Can you work these out from the model? Positions are in its coordinate system, mm. A direction names the side the tool comes from. Coordinates: 2 decimals unless noted, no trailing zeros. Loops run counter-clockwise (first coordinate to the right, second up) from the corner with the lowest first, then second, coordinate; pieces in that order, holes last. Notation, with made-up numbers: M 55.25,63 L 87.25,63 A21 cw 87.25,96 Z; hole C -12,5.25 d8. An arc over 180 degrees is marked long. Answer as a JSON object with one key per item and string values. Group by question number.
Item 1: Suppose I cut it at C-C (z = -3.5). Write out the boundary of the cut face in (x, y), then the cut area to 3 significant figures.
Item 2: Suppose I cut it at A-A (y = 2.5). Write out the boundary of the cut face in (x, z).
Item 3: Suppose I cut it at B-B (x = 3). Write out the boundary of the cut face in (y, z).
Item 4: We'd pull the mould along Y, two halves only. Please class faces 3 (the flat face through (3, 9, -3)), 4 (the flat face through (6, 5, -3)), 5 (the cylindrical face through (5.49, 2.88, -4.69)): +Y half, -Y half, draft (parallel to the pull), parting line (faces both ways), or undercut.
Item 5: I'm going to push flat-ended pins straight in: pin 1 Ø1.2 at (x, y) = (4, 2) entering from -Z; pin 2 Ø2 at (x, z) = (5.5, -3.5) entering from -Y. Where does each tip first touch, or does it pass through?
Item 6: Which directions (+Z, -Z, +X, -X, +Y, -Y) give clear straight access to the entire face, cutting with the end or side of a thin tool? Please do faces 1 (the flat face through (5, 3, -2)), 2 (the cylindrical face through (1.23, 0.46, -5.02)).
Item 7: Suppose I cut it at D-D (y = 7). Write out the boundary of the cut face in (x, z), then the cut area to 3 significant figures.
Item 8: If I drill on line 1 (X direction, y = 0.75, z = -2.8); line 2 (Y direction, x = 0.5, z = -3.5); line 3 (Z direction, x = 1.2, y = 2.5), over which ranges is the centre line in solid material (lowest first)?
```python
from build123d import *

# Parameters (mm, degrees)
SKETCH1_W           = 5.5
SKETCH1_H           = 9
SKETCH1_R           = 1.25
BOSS_EXTRUDE1_DEPTH = 6
CUT_EXTRUDE3_DEPTH  = 4.5
CUT_EXTRUDE4_REACH  = 14.135
SKETCH5_R           = 1.25
FILLET1_R           = 1.6


with BuildPart() as part:
    # Sketch1 → Boss-Extrude1 (new body)
    with BuildSketch(Plane(origin=(0, 0, 0), x_dir=(0, 0, -1), z_dir=(1, 0, 0))):
        with Locations((2.75, 4.5)):
            Rectangle(SKETCH1_W, SKETCH1_H)
        with Locations((3.5, 2.5)):
            Circle(SKETCH1_R, mode=Mode.SUBTRACT)
    extrude(amount=BOSS_EXTRUDE1_DEPTH)

    # Sketch4 → Cut-Extrude3 (cut)
    with BuildSketch(Plane(origin=(0, 0, -5.5), x_dir=(-1, 0, 0), z_dir=(0, 0, -1))):
        with BuildLine():
            Line((-5, 0), (-5, 4.8))
            ThreePointArc((-5, 4.8), (-3.75, 6.05), (-2.5, 4.8))
            Line((-2.5, 4.8), (-2.5, 0))
            ThreePointArc((-2.5, 0), (-3.75, -1.25), (-5, 0))
        make_face()
    extrude(amount=-CUT_EXTRUDE3_DEPTH, mode=Mode.SUBTRACT)

    # Sketch5 → Cut-Extrude4 (cut, up to next)
    with BuildSketch(Plane.ZY, mode=Mode.PRIVATE) as cut_extrude4_sk1:
        with Locations((-3, 7)):
            Circle(SKETCH5_R)
    cut_extrude4_tool1 = extrude(cut_extrude4_sk1.sketch, amount=-CUT_EXTRUDE4_REACH, mode=Mode.PRIVATE) & part.part
    add(cut_extrude4_tool1.solids().sort_by_distance((0, 7, -3))[0], mode=Mode.SUBTRACT)

    # Fillet1
    # the kernel refuses this fillet: 1.6 mm, written as the material it takes off along each edge
    with BuildSketch(Plane(origin=(-4, 0, 0), x_dir=(0, 0, -1), z_dir=(1, 0, 0)), Plane(origin=(-4, 9, 0), x_dir=(0, -1, 0), z_dir=(1, 0, 0))) as fillet1_piece_1:
        with BuildLine():
            CenterArc((FILLET1_R, FILLET1_R), FILLET1_R, 180, 90)
            Line((0, FILLET1_R), (0, 0))
            Line((0, 0), (FILLET1_R, 0))
        make_face()
    extrude(amount=14, mode=Mode.SUBTRACT)
    with BuildSketch(Plane(origin=(1, 0, -5.5), x_dir=(0, 0, 1), z_dir=(1, 0, 0))) as fillet1_piece_2:
        with BuildLine():
            CenterArc((FILLET1_R, -FILLET1_R), FILLET1_R, 90, 90)
            Line((0, -FILLET1_R), (0, 0))
            Line((0, 0), (FILLET1_R, 0))
        make_face()
    extrude(amount=9, mode=Mode.SUBTRACT)
    with BuildSketch(Plane(origin=(-4, 0, -5.5), x_dir=(0, 0, 1), z_dir=(1, 0, 0))) as fillet1_piece_3:
        with BuildLine():
            CenterArc((FILLET1_R, -FILLET1_R), FILLET1_R, 90, 90)
            Line((0, -FILLET1_R), (0, 0))
            Line((0, 0), (FILLET1_R, 0))
        make_face()
    extrude(amount=10.5, mode=Mode.SUBTRACT)
    with BuildSketch(Plane(origin=(-4, 9, -5.5), x_dir=(0, -1, 0), z_dir=(1, 0, 0))) as fillet1_piece_4:
        with BuildLine():
            CenterArc((FILLET1_R, -FILLET1_R), FILLET1_R, 90, 90)
            Line((0, -FILLET1_R), (0, 0))
            Line((0, 0), (FILLET1_R, 0))
        make_face()
    extrude(amount=14, mode=Mode.SUBTRACT)


solid = part.part
```
From the geometry:
{
 "1": {"outline": "M 0,0 L 2.5,0 L 2.5,1.25 L 0,1.25 Z; M 0,3.75 L 2.5,3.75 L 2.5,4.8 A1.25 cw 3.08,5.85 L 0,5.85 Z; M 0,8.15 L 6,8.15 L 6,9 L 0,9 Z; M 4.42,5.85 A1.25 cw 5,4.8 L 5,3.75 L 6,3.75 L 6,5.85 Z; M 5,0 L 6,0 L 6,1.25 L 5,1.25 Z", "area": "17.2 mm2"},
 "2": {"outline": "M 0,-5.5 L 2.5,-5.5 L 2.5,-4.75 L 0,-4.75 Z; M 0,-2.25 L 2.5,-2.25 L 2.5,-1 L 5,-1 L 5,-2.25 L 6,-2.25 L 6,0 L 0,0 Z; M 5,-5.5 L 6,-5.5 L 6,-4.75 L 5,-4.75 Z"},
 "3": {"outline": "M 0.12,-1 L 5.8,-1 L 5.8,-2.65 A1.25 cw long 5.8,-3.35 L 5.8,-5.5 L 7.4,-5.5 A1.6 ccw 9,-3.9 L 9,-1.6 A1.6 ccw 7.4,0 L 1.6,0 A1.6 ccw Z"},
 "4": {"face 3": "+Y half", "face 4": "draft", "face 5": "undercut"},
 "5": {"pin 1": "z = -1", "pin 2": "y = 0"},
 "6": {"face 1": "-Z, -Y", "face 2": "-Z, +X, -X, -Y"},
 "7": {"outline": "M 0,-5.5 L 6,-5.5 L 6,-4.25 L 0,-4.25 Z; M 0,-1.75 L 6,-1.75 L 6,0 L 0,0 Z", "area": "18.0 mm2"},
 "8": {"line 1": "0 to 2.5, 5 to 6", "line 2": "0 to 1.25, 3.75 to 5.85, 8.15 to 9", "line 3": "-5.5 to -4.75, -2.25 to 0"}
}
